Autodesk Inventor part; units mm, degrees
ref_plane "YZ Plane" through (0, 0, 0) normal (1, 0, 0) x (0, 1, 0)
ref_plane "XZ Plane" through (0, 0, 0) normal (0, 1, 0) x (-1, 0, 0)
ref_plane "XY Plane" through (0, 0, 0) normal (0, 0, 1) x (1, 0, 0)
sketch "Boceto39" plane through (0, 0, 0) normal (0, 0, 1) x (1, 0, 0)
  circle A0 centre (0, -1.27) radius 0.25
  circle A1 centre (5.08, 1.27) radius 0.25
  circle A2 centre (-7.62, 1.27) radius 0.25
  point P0 (0, 0)
  dimension "d373" = 0.5
  dimension "d376" = 12.7
  dimension "d377" = 5.08
  dimension "d392" = 1.27
  dimension "d393" = 2.54
extrude "Extrusión13" add sketch "Boceto39" against normal blind 2.6
sketch "Boceto40" plane through (0, 0, 0) normal (0, 0, 1) x (1, 0, 0)
  line L0 (-11.3, 2.5) -> (8, 2.5)
  line L1 (8, 2.5) -> (8, -2.5)
  line L2 (8, -2.5) -> (-11.3, -2.5)
  line L3 (-11.3, -2.5) -> (-11.3, 2.5)
  point P0 (0, 0)
  point P1 (8, 0)
  dimension "d380" = 5
  dimension "d381" = 19.3
  dimension "d382" = 8
extrude "Extrusión14" add sketch "Boceto40" along normal blind 7
sketch "Boceto41" plane through (8, -2.5, 0) normal (1, 0, 0) x (0, 0, -1)
  circle A0 centre (-5.1, 2.5) radius 1.2
  line L0 (-7, 0) -> (-7, 5)
  line L1 (0, 5) -> (0, 0)
  point P0 (0, 2.5)
  point P1 (0, 2.5)
  dimension "d385" = 2.4
  dimension "d386" = 1.9
extrude "Extrusión15" add sketch "Boceto41" along normal blind 1.2
sketch "Boceto42" plane through (9.2, 0, 5.1) normal (1, 0, 0) x (0, 0, -1)
  line L0 (-1.4485, 0.3) -> (1.5656, 0.3)
  line L1 (1.5656, 0.3) -> (1.5656, -0.3)
  line L2 (1.5656, -0.3) -> (-1.4485, -0.3)
  line L3 (-1.4485, -0.3) -> (-1.4485, 0.3)
  point P0 (5.1, 0)
  point P1 (1.5656, 0)
  dimension "d389" = 0.6
extrude "Extrusión16" cut sketch "Boceto42" against normal blind 0.5
properties part number "RES-PRESET-3006P"
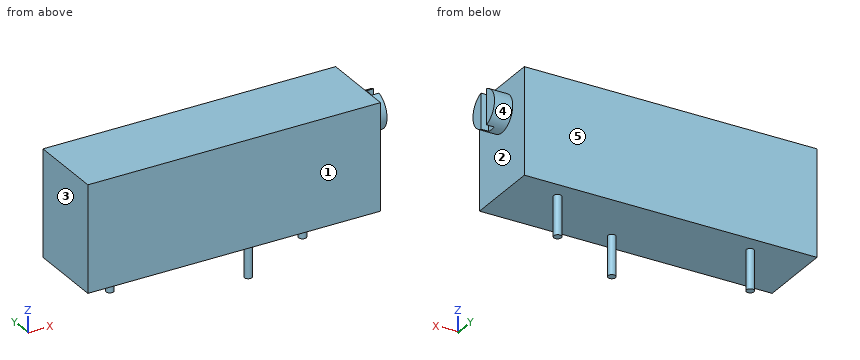
Here's how the part is built. I have some questions about the finished solid (model axes, mm). Face numbers are marked on the shaded views. A direction names the side the tool comes from. Give positions to 0.01 mm unless a question says otherwise; leave off trailing zeros. Order: outer loops, then holes, each group sorted by start corner. A loop starts at its lowest first (then second) coordinate and runs counter-clockwise, first axis right, second up. Notation, with made-up numbers: (87.5, 7.25) - (139.5, 7.25) arc R21 ccw to (139.5, 14.25) - close; hole circle Ø8 at (85, 74). An arc over 180 degrees is marked (long way). Answer as a JSON object with one key per item and string values. Group by question number.
Item 1: If we section it at C-C on z = 4.75: Please give me the cut outline in (x, y).
Item 2: If we section it at B-B on y = 0: Please give me the cut outline in (x, z).
Item 3: If we mould it in two halves opening along X, with no side actions, what happens to the marked faces 1, 2 and 3? For each: pulls with the +X half, pulls with the -X half, needs draft (parallel to the pull), parting line crosses it, or undercut.
Item 4: For P1, Ø0.6, axis at x = 9, z = 5, coming from the +Y side, with a flat end and sliding along its axis, tell me the tip position at first contact or that it passes through.
Item 5: Please list where these lines run through material, in increasing order: probe 1 along Z at (x, y) = (-1, 1.55); probe 2 along X at (y, z) = (2.05, 4.5).
Item 6: If we section it at D-D on z = 1: Please give me the cut outline in (x, y).
Item 7: If we section it at A-A on x = 5.08: Please give me the cut outline in (y, z), and give its area (3 significant figures).
Item 8: Which directions (+Z, -Z, +X, -X, +Y, -Y) give clear straight access to the entire face, cutting with the end or side of a thin tool? Please do the marked faces 4 and 5.
Result set:
{
 "1": {"outline": "(-11.3, -2.5) - (8, -2.5) - (8, -1.15) - (9.2, -1.15) - (9.2, -0.3) - (8.7, -0.3) - (8.7, 0.3) - (9.2, 0.3) - (9.2, 1.15) - (8, 1.15) - (8, 2.5) - (-11.3, 2.5) - close"},
 "2": {"outline": "(-11.3, 0) - (8, 0) - (8, 3.9) - (8.7, 3.9) - (8.7, 6.3) - (8, 6.3) - (8, 7) - (-11.3, 7) - close"},
 "3": {"face 1": "needs draft", "face 2": "pulls with the +X half", "face 3": "pulls with the -X half"},
 "4": {"P1": "y = 1.2"},
 "5": {"probe 1": "0 to 7", "probe 2": "-11.3 to 8"},
 "6": {"outline": "(-11.3, -2.5) - (8, -2.5) - (8, 2.5) - (-11.3, 2.5) - close"},
 "7": {"outline": "(-2.5, 0) - (1.02, 0) - (1.02, -2.6) - (1.52, -2.6) - (1.52, 0) - (2.5, 0) - (2.5, 7) - (-2.5, 7) - close", "area": "36.3 mm²"},
 "8": {"face 4": "+X", "face 5": "+Z, -Z, +X, -X, +Y"}
}
